Verification items for the finished model (mm, model axes). A direction names the side the tool comes from. Give positions to 0.01 mm unless a question says otherwise; leave off trailing zeros. Loops run counter-clockwise (first coordinate to the right, second up) from the corner with the lowest first, then second, coordinate; pieces in that order, holes last. Notation, with made-up numbers: (-0.5, 36) - (24.5, 36) arc R5 ccw to (24.5, 43) - close; hole circle Ø10 at (45, -30). An arc over 180 degrees is marked (long way). Use one line per item in the form item = value.
```python
from build123d import *

# Parameters (mm, degrees)
F0_R     = 12.7
F1_DEPTH = 25.4
F2_R     = 12.7
F3_DEPTH = 25.4
F4_DEPTH = 25.4
F5_DEPTH = 25.4
F6_R     = 12.7


with BuildPart() as f1:
    # F0 (on Front) → F1 (new body)
    with BuildSketch(Plane.XZ):
        with BuildLine():
            Line((61.959432, -7.667416), (-25.402695, 51.466912))
            ThreePointArc((-25.402695, 51.466912), (-51.546828, 52.869183), (-65.040568, 30.432584))
            Line((-65.040568, 30.432584), (-65.040568, -20.367416))
            Line((-65.040568, -20.367416), (61.959432, -20.367416))
            Line((61.959432, -20.367416), (61.959432, -7.667416))
        make_face()
        with Locations((-39.640568, 30.432584)):
            Circle(F0_R, mode=Mode.SUBTRACT)
    extrude(amount=F1_DEPTH)

    # F2 (on face) → F3 (join)
    with BuildSketch(Plane.XZ.offset(25.4)):
        with BuildLine():
            ThreePointArc((-14.240568, 30.432584), (-17.203969, 42.338843), (-25.402695, 51.466912))
            ThreePointArc((-25.402695, 51.466912), (-51.546828, 52.869183), (-65.040568, 30.432584))
            ThreePointArc((-65.040568, 30.432584), (-40.000603, 5.035136), (-14.250775, 29.712586))
            ThreePointArc((-14.250775, 29.712586), (-14.24312, 30.072549), (-14.240568, 30.432584))
        make_face()
        with Locations((-39.640568, 30.432584)):
            Circle(F2_R, mode=Mode.SUBTRACT)
    extrude(amount=F3_DEPTH)

    # F2 (on face) → F4 (join)
    with BuildSketch(Plane.XZ.offset(25.4)):
        with BuildLine():
            ThreePointArc((-14.240568, 30.432584), (-17.203969, 42.338843), (-25.402695, 51.466912))
            ThreePointArc((-25.402695, 51.466912), (-51.546828, 52.869183), (-65.040568, 30.432584))
            ThreePointArc((-65.040568, 30.432584), (-40.000603, 5.035136), (-14.250775, 29.712586))
            ThreePointArc((-14.250775, 29.712586), (-14.24312, 30.072549), (-14.240568, 30.432584))
        make_face()
        with Locations((-39.640568, 30.432584)):
            Circle(F2_R, mode=Mode.SUBTRACT)
    extrude(amount=F4_DEPTH)

    # F2 (on face) → F5 (join)
    with BuildSketch(Plane.XZ.offset(25.4)):
        with BuildLine():
            Line((61.959432, -20.367416), (61.959432, -7.667416))
            Line((61.959432, -7.667416), (-14.250775, -7.667416))
            Line((-14.250775, -7.667416), (-14.250775, 29.712586))
            ThreePointArc((-14.250775, 29.712586), (-40.000603, 5.035136), (-65.040568, 30.432584))
            Line((-65.040568, 30.432584), (-65.040568, -7.667416))
            Line((-65.040568, -7.667416), (-65.040568, -20.367416))
            Line((-65.040568, -20.367416), (61.959432, -20.367416))
        make_face()
        with BuildLine():
            ThreePointArc((-14.240568, 30.432584), (-17.203969, 42.338843), (-25.402695, 51.466912))
            ThreePointArc((-25.402695, 51.466912), (-51.546828, 52.869183), (-65.040568, 30.432584))
            ThreePointArc((-65.040568, 30.432584), (-40.000603, 5.035136), (-14.250775, 29.712586))
            ThreePointArc((-14.250775, 29.712586), (-14.24312, 30.072549), (-14.240568, 30.432584))
        make_face()
        with Locations((-39.640568, 30.432584)):
            Circle(F2_R, mode=Mode.SUBTRACT)
    extrude(amount=F5_DEPTH)

    # F6
    f6_edges = [f1.edges().sort_by_distance(p)[0] for p in [
        (61.959432, -50.8, -14.017416),
    ]]
    fillet(f6_edges, radius=F6_R)


solid = f1.part
```
1. Draft check along Z on faces 1 (the flat face through (-17, 0, 10)), 2 (the cylindrical face through (-49.719, -25.044, 22.705)), 3 (the flat face through (24, -38, -7.667)), 4 (the flat face through (-2, -25, -20.367)). Enter one of: released by +Z, released by -Z, zero draft, split by the parting line, or undercut.
Result set:
face_1 = zero draft
face_2 = undercut
face_3 = released by +Z
face_4 = released by -Z
2. Depth check by flat-ended pin: pin 1 Ø12 at (x, y) = (-41.5, -16) entering from +Z; pin 2 Ø15 at (x, z) = (-39.64, 30.43) entering from +Y; pin 3 Ø12.5 at (y, z) = (-43.5, 12.5) entering from +X; pin 4 Ø10 at (x, z) = (-9, 1.5) entering from -Y. Enter the tip coordinate at first touch or a pass-through.
Result set:
pin_1 = 55.83
pin_2 = through
pin_3 = -14.25
pin_4 = -25.4
3. Section check D-D, the plane y = -9. Record the cut outline in (x, z), then the cut area to 3 significant figures.
Result set:
outline = (-65.04, -20.37) - (61.96, -20.37) - (61.96, -7.67) - (-25.4, 51.47) arc R25.4 ccw to (-65.04, 30.43) - close; hole circle Ø25.4 at (-39.64, 30.43)
area = 6,050 mm²
4. Tool access check on faces 5 (the flat face through (61.959, -19, -14)), 6 (the flat face through (-14.251, -38, 11)). Record the directions out of +Z, -Z, +X, -X, +Y, -Y that give a thin tool (end or side, any length) a straight path to the whole face; none if there is none.
Result set:
face_5 = +Z, -Z, +X, +Y, -Y
face_6 = +Z, +X, -Y
5. Section check A-A, the plane y = -31.5. Record the cut outline in (x, z), then the cut area to 3 significant figures.
Result set:
outline = (-65.04, -20.37) - (61.96, -20.37) - (61.96, -7.67) - (-14.25, -7.67) - (-14.25, 29.71) arc R25.4 ccw to (-14.24, 30.43) arc R25.4 ccw to (-25.4, 51.47) arc R25.4 ccw to (-65.04, 30.43) - close; hole circle Ø25.4 at (-39.64, 30.43)
area = 4,050 mm²
6. Section check C-C, the plane z = 37. Record the cut outline in (x, y), then the cut area to 3 significant figures.
Result set:
outline = (-64.18, -50.8) - (-50.51, -50.8) - (-50.51, 0) - (-64.18, 0) - close; (-28.77, -50.8) - (-15.1, -50.8) - (-15.1, -25.4) - (-4.03, -25.4) - (-4.03, 0) - (-28.77, 0) - close
area = 1,670 mm²
7. Scan lines: probe 1 along Z at (x, y) = (10.5, -42); probe 2 along X at (y, z) = (-26, 38); probe 3 along X at (y, z) = (-6.5, 25.5). Record each from-to range of solid material in increasing order.
Result set:
probe_1 = -20.37 to -7.67
probe_2 = -63.89 to -49.84, -29.44 to -15.39
probe_3 = -65.04 to -51.34, -27.94 to 12.96
8. Section check B-B, the plane x = -31. Record the cut outline in (y, z), then the cut area to 3 significant figures.
Result set:
outline = (-50.8, -20.37) - (0, -20.37) - (0, 21.13) - (-50.8, 21.13) - close; (-50.8, 39.74) - (0, 39.74) - (0, 54.32) - (-50.8, 54.32) - close
area = 2,850 mm²
